```python
from build123d import *

# Parameters (mm, degrees)
SKETCH2_W           = 84.57
SKETCH2_H           = 90.8
BOSS_EXTRUDE1_DEPTH = 1.6
SKETCH3_R           = 1.5
CUT_EXTRUDE1_DEPTH  = 2.6
SKETCH4_W           = 90.8
SKETCH4_H           = 1.6
BOSS_EXTRUDE2_DEPTH = 2.88
SKETCH5_W           = 90.8
SKETCH5_H           = 1.6
BOSS_EXTRUDE3_DEPTH = 2.59
SKETCH6_W           = 90.04
SKETCH6_H           = 1.6
BOSS_EXTRUDE4_DEPTH = 2.54
SKETCH7_W           = 90.04
SKETCH7_H           = 1.6
BOSS_EXTRUDE5_DEPTH = 2.54
SKETCH8_W           = 16.372642976
SKETCH8_H           = 45.571517242
SKETCH8_W_2         = 42.266473234
SKETCH8_H_2         = 21.901065616
SKETCH8_W_3         = 18.617013656
SKETCH8_H_3         = 45.520108402
SKETCH8_W_4         = 42.118702304
SKETCH8_H_4         = 22.400138828
CUT_EXTRUDE2_DEPTH  = 2.6


with BuildPart() as part:
    # Sketch2 → Boss-Extrude1 (new body)
    with BuildSketch(Plane(origin=(0, 0, 0), x_dir=(1, 0, 0), z_dir=(0, 1, 0))):
        with Locations((42.285, 45.4)):
            Rectangle(SKETCH2_W, SKETCH2_H)
    extrude(amount=BOSS_EXTRUDE1_DEPTH)

    # Sketch3 → Cut-Extrude1 (cut, through all)
    with BuildSketch(Plane(origin=(0, 1.6, 0), x_dir=(1, 0, 0), z_dir=(0, 1, 0))):
        with Locations((2.5, 2.5)):
            Circle(SKETCH3_R)
        with Locations((82.07, 2.5)):
            Circle(SKETCH3_R)
        with Locations((5.8, 88.3)):
            Circle(SKETCH3_R)
        with Locations((79.37, 88.3)):
            Circle(SKETCH3_R)
    extrude(amount=-CUT_EXTRUDE1_DEPTH, mode=Mode.SUBTRACT)

    # Sketch4 → Boss-Extrude2 (add)
    with BuildSketch(Plane(origin=(84.57, 0, 0), x_dir=(0, 0, -1), z_dir=(1, 0, 0))):
        with Locations((45.4, 0.8)):
            Rectangle(SKETCH4_W, SKETCH4_H)
    extrude(amount=BOSS_EXTRUDE2_DEPTH)

    # Sketch5 → Boss-Extrude3 (add)
    with BuildSketch(Plane.ZY):
        with Locations((-45.4, 0.8)):
            Rectangle(SKETCH5_W, SKETCH5_H)
    extrude(amount=BOSS_EXTRUDE3_DEPTH)

    # Sketch6 → Boss-Extrude4 (add)
    with BuildSketch(Plane(origin=(0, 0, -90.8), x_dir=(-1, 0, 0), z_dir=(0, 0, -1))):
        with Locations((-42.43, 0.8)):
            Rectangle(SKETCH6_W, SKETCH6_H)
    extrude(amount=BOSS_EXTRUDE4_DEPTH)

    # Sketch7 → Boss-Extrude5 (add)
    with BuildSketch(Plane.XY):
        with Locations((42.43, 0.8)):
            Rectangle(SKETCH7_W, SKETCH7_H)
    extrude(amount=BOSS_EXTRUDE5_DEPTH)

    # Sketch8 → Cut-Extrude2 (cut, through all)
    with BuildSketch(Plane(origin=(0, 1.6, 0), x_dir=(1, 0, 0), z_dir=(0, 1, 0))):
        with Locations((87.45, 45.4)):
            Rectangle(SKETCH8_W, SKETCH8_H)
        with Locations((42.43, 93.34)):
            Rectangle(SKETCH8_W_2, SKETCH8_H_2)
        with Locations((-2.59, 45.4)):
            Rectangle(SKETCH8_W_3, SKETCH8_H_3)
        with Locations((42.43, -2.54)):
            Rectangle(SKETCH8_W_4, SKETCH8_H_4)
    extrude(amount=-CUT_EXTRUDE2_DEPTH, mode=Mode.SUBTRACT)


solid = part.part
```
Could you check a few things on this model? Use its own coordinates, in mm. Give positions to 0.01 mm unless a question says otherwise; leave off trailing zeros. Loops run counter-clockwise (first coordinate to the right, second up) from the corner with the lowest first, then second, coordinate; pieces in that order, holes last. Notation, with made-up numbers: (64.25, -16) -> (80.25, -16) arc R28 ccw to (80.25, 14) -> close; hole circle Ø1 at (44.25, 52). An arc over 180 degrees is marked (long way). Put each result on its own line as item: value.
(1) Imagine slicing it at C-C on y = 0.35. Write out the boundary of the cut face in (x, z).
Computed:
outline: (-2.59, -93.34) -> (21.3, -93.34) -> (21.3, -82.39) -> (63.56, -82.39) -> (63.56, -93.34) -> (87.45, -93.34) -> (87.45, -68.19) -> (79.26, -68.19) -> (79.26, -22.61) -> (87.45, -22.61) -> (87.45, 2.54) -> (63.49, 2.54) -> (63.49, -8.66) -> (21.37, -8.66) -> (21.37, 2.54) -> (-2.59, 2.54) -> (-2.59, -22.64) -> (6.72, -22.64) -> (6.72, -68.16) -> (-2.59, -68.16) -> close; hole circle Ø3 at (2.5, -2.5); hole circle Ø3 at (5.8, -88.3); hole circle Ø3 at (79.37, -88.3); hole circle Ø3 at (82.07, -2.5)
(2) Imagine slicing it at A-A on z = -88.3. Write out the boundary of the cut face in (x, y).
Computed:
outline: (-2.59, 0) -> (4.3, 0) -> (4.3, 1.6) -> (-2.59, 1.6) -> close; (7.3, 0) -> (21.3, 0) -> (21.3, 1.6) -> (7.3, 1.6) -> close; (63.56, 0) -> (77.87, 0) -> (77.87, 1.6) -> (63.56, 1.6) -> close; (80.87, 0) -> (87.45, 0) -> (87.45, 1.6) -> (80.87, 1.6) -> close
(3) Imagine slicing it at D-D on z = -6.5. Write out the boundary of the cut face in (x, y), plus the area to 3 significant figures.
Computed:
outline: (-2.59, 0) -> (21.37, 0) -> (21.37, 1.6) -> (-2.59, 1.6) -> close; (63.49, 0) -> (87.45, 0) -> (87.45, 1.6) -> (63.49, 1.6) -> close
area: 76.7 mm^2
(4) I'm going to push flat-ended pins straight in: pin 1 Ø0.5 at (x, y) = (49, 1) entering from +Z; pin 2 Ø0.8 at (y, z) = (0.5, -45) entering from -X; pin 3 Ø4 at (x, z) = (5.8, -88.3) entering from -Y; pin 4 Ø2.5 at (x, z) = (82.07, -2.5) entering from -Y. Where does each tip first touch, or does it pass through?
Computed:
pin 1: z = -8.66
pin 2: x = 6.72
pin 3: y = 0
pin 4: through
(5) Thinking about a two-plate mould opening in X: for faces 1 (the face through (42, 1.6, -46)), 2 (the face through (2.175, 0.811, -1.036)), which applies, pulls with the +X half, pulls with the -X half, needs draft (parallel to the pull), parting line crosses it, or undercut?
Computed:
face 1: needs draft
face 2: undercut
(6) Please list where these lines run through material, in increasing order: probe 1 along Z at (x, y) = (2.5, 1.05); probe 2 along X at (y, z) = (0.9, -2.5); probe 3 along Z at (x, y) = (5.8, 1.2). Write a range as [from, to].
Computed:
probe 1: [-93.34, -68.16], [-22.64, -4], [-1, 2.54]
probe 2: [-2.59, 1], [4, 21.37], [63.49, 80.57], [83.57, 87.45]
probe 3: [-93.34, -89.8], [-86.8, -68.16], [-22.64, 2.54]
(7) Imagine slicing it at B-B on x = 82.07. Write out the boundary of the cut face in (y, z), plus the area to 3 significant figures.
Computed:
outline: (0, -93.34) -> (1.6, -93.34) -> (1.6, -68.19) -> (0, -68.19) -> close; (0, -22.61) -> (1.6, -22.61) -> (1.6, -4) -> (0, -4) -> close; (0, -1) -> (1.6, -1) -> (1.6, 2.54) -> (0, 2.54) -> close
area: 75.7 mm^2
